from build123d import *

# Parameters (mm, degrees)
SKETCH040_W    = 250
SKETCH040_H    = 268
PAD011_DEPTH   = 55
FILLET013_R    = 6
THICKNESS001_T = 3


with BuildPart() as part:
    # Sketch040 → Pad011 (new body)
    with BuildSketch(Plane.XY):
        with Locations((0, -134)):
            Rectangle(SKETCH040_W, SKETCH040_H)
    extrude(amount=PAD011_DEPTH)

    # Fillet013
    fillet013_edges = [part.edges().sort_by_distance(p)[0] for p in [
        (125, -268, 27.5),
        (-125, -268, 27.5),
    ]]
    fillet(fillet013_edges, radius=FILLET013_R)

    # Thickness001
    thickness001_openings = [part.faces().sort_by_distance(p)[0] for p in [
        (0, -133.969399, 55),
        (0, -133.969399, 0),
        (0, 0, 27.5),
    ]]
    offset(amount=THICKNESS001_T, openings=thickness001_openings)


solid = part.part
For this review, take the finished solid that the model builds, in its own axes (mm). A direction names the side the tool comes from. Round coordinates to 2 decimals unless told otherwise and drop trailing zeros. Order: outer loops, then holes, each group sorted by start corner. A loop starts at its lowest first (then second) coordinate and runs counter-clockwise, first axis right, second up. Notation, with made-up numbers: M 19.25,-11.75 L 65.25,-11.75 A29 cw 65.25,21.25 Z; hole C -14.75,27 d4. An arc over 180 degrees is marked long. Use a Markdown table: item, result. Add a question column.
Item 1: To check wall thickness, follow line 1 along X through (y, z) = (-17, 4.5); line 2 along Y through (x, z) = (-77.5, 52). State the ranges of each line that lie inside material, in increasing order.
Item 2: Mouldability with a two-part tool opening along X and no side actions: class faces 1 (the cylindrical face through (-123.289, -266.196, 27.885)), 2 (the flat face through (128, -133, 27)), 3 (the flat face through (-128, -133, 27)) as released by +X, released by -X, zero draft, split by the parting line, or undercut.
Item 3: Add section C-C, the plane x = 104. Give the boundary of the cut face in (y, z).
Item 4: Tool access review of faces 4 (the flat face through (-2, -271, 27)), 5 (the flat face through (-2, -268, 27)): name each direction out of +Z, -Z, +X, -X, +Y, -Y from which nothing blocks a thin tool from reaching the whole face with its end or side.
Item 5: Insertion check: pin 1 (8 mm diameter, centred on x = 15, z = 38, fed in from +Y). The pin has a flat end and moves straight along its axis. Give the tip position at first contact, or say it passes through.
Item 6: Add section B-B, the plane z = 12. Give the boundary of the cut face in (x, y), then the cut area to 3 significant figures.
Item 7: Add section A-A, the plane y = -242. Give the boundary of the cut face in (x, z).
Geometry results:
| question | item | result |
|---|---|---|
| 1 | line 1 | x = -128 to -125, 125 to 128 |
| 1 | line 2 | y = -271 to -268 |
| 2 | face 1 | undercut |
| 2 | face 2 | released by +X |
| 2 | face 3 | released by -X |
| 3 | outline | M -271,0 L -268,0 L -268,55 L -271,55 Z |
| 4 | face 4 | +Z, -Z, +X, -X, -Y |
| 4 | face 5 | +Z, -Z, +Y |
| 5 | pin 1 | stops at y = -268 |
| 6 | outline | M -128,-262 A9 ccw -119,-271 L 119,-271 A9 ccw 128,-262 L 128,0 L 125,0 L 125,-262 A6 cw 119,-268 L -119,-268 A6 cw -125,-262 L -125,0 L -128,0 Z |
| 6 | area | 2,360 mm² |
| 7 | outline | M -128,0 L -125,0 L -125,55 L -128,55 Z; M 125,0 L 128,0 L 128,55 L 125,55 Z |
